Input: part model. Units: mm. Frame: model coordinates. A direction names the side the tool comes from. Coordinates: 2 decimals unless noted, no trailing zeros. Write each loop counter-clockwise with the first axis right and the second up, starting at its lowest first coordinate (ties: lowest second). Pieces come first, ordered by that corner, then holes. Notation, with made-up numbers: (69, -21.75) - (125, -21.75) arc R15 ccw to (125, 2.25) - close; hole circle Ø9 at (64, 81.25). An arc over 180 degrees is marked (long way). Put each result on its own line as item: value. Start each with the question number.
1. Cut plane D-D, the plane x = 29.5. Return loops of the section in (y, z).
2. Cut plane C-C, the plane x = 48. Return loops of the section in (y, z), and give its area (3 significant figures).
3. Line query: line 1 (Z direction, x = 3, y = -29.5); line 2 (X direction, y = -18.5, z = -20.5); line 3 (X direction, y = -7, z = 3). Output: solid intervals per line, ascending.
4. Pin query (flat end, axial travel): pin 1 (5.5 mm diameter, centred on y = -7.5, z = 13, fed in from -X); pin 2 (1.5 mm diameter, centred on y = -16.5, z = 7, fed in from +X); pin 3 (6 mm diameter, centred on x = 35, y = -9.5, fed in from +Z). Return the tip coordinate at first contact, or that it passes through.
5. Cut plane A-A, the plane z = 14. Return loops of the section in (x, y).
6. Pull-direction query (X, two-part tool) for faces 5 (the flat face through (43.25, -9.392, 7.054)), 6 (the flat face through (9, -19, -40.078)), 7 (the flat face through (-20.52, -9.39, 7.19)); classes: released by +X, released by -X, zero draft, split by the parting line, or undercut.
7. Cut plane B-B, the plane y = -12.5. Return loops of the section in (x, z).
8. Access query for faces 1 (the flat face through (-53.153, -19, -24)), 2 (the flat face through (11.055, -9, 8)), 3 (the flat face through (-35, -19.05, 1)), 4 (the flat face through (-52.445, -9, 8)). Directions: +Z, -Z, +X, -X, +Y, -Y. A direction counts if a zero-diameter tool reaches every point of the face in a straight line with its end or side. Return the directions, or none.
from build123d import *

# Parameters (mm, degrees)
F0_W     = 127
F0_H     = 31.75
F1_DEPTH = 38.1
F3_DEPTH = 19.05


with BuildPart() as f1:
    # F0 (on Front) → F1 (new body)
    with BuildSketch(Plane.XZ):
        with Locations((10.347378, -24.202869)):
            Rectangle(F0_W, F0_H)
    extrude(amount=F1_DEPTH)

    # F2 (on Front) → F3 (join)
    with BuildSketch(Plane.XZ):
        Polygon((-52.444755, 23.151476), (-52.444755, -8.598524), (11.055245, -8.598524), align=None)
        Polygon((11.055245, 23.151476), (11.055245, -8.598524), (74.555245, -8.598524), align=None)
    extrude(amount=F3_DEPTH)


solid = f1.part
Report:
1. outline: (-38.1, -40.08) - (0, -40.08) - (0, 13.93) - (-19.05, 13.93) - (-19.05, -8.33) - (-38.1, -8.33) - close
2. outline: (-38.1, -40.08) - (0, -40.08) - (0, 4.68) - (-19.05, 4.68) - (-19.05, -8.33) - (-38.1, -8.33) - close
2. area: 1,460 mm^2
3. line 1: z = -40.08 to -8.33
3. line 2: x = -53.15 to 73.85
3. line 3: x = -52.44 to -12.14, 11.06 to 51.36
4. pin 1: stops at x = -52.44
4. pin 2: stops at x = 44.86
4. pin 3: stops at z = 12.68
5. outline: (-52.44, -19.05) - (-34.14, -19.05) - (-34.14, 0) - (-52.44, 0) - close; (11.06, -19.05) - (29.36, -19.05) - (29.36, 0) - (11.06, 0) - close
6. face 5: released by +X
6. face 6: zero draft
6. face 7: undercut
7. outline: (-53.15, -40.08) - (73.85, -40.08) - (73.85, -8.6) - (74.56, -8.6) - (11.06, 23.15) - (11.06, -8.33) - (10.51, -8.33) - (-52.44, 23.15) - (-52.44, -8.33) - (-53.15, -8.33) - close
8. face 1: +Z, -Z, -X, +Y, -Y
8. face 2: +Z, +Y, -Y
8. face 3: +Z, +X, -X, -Y
8. face 4: +Z, -X, +Y, -Y
